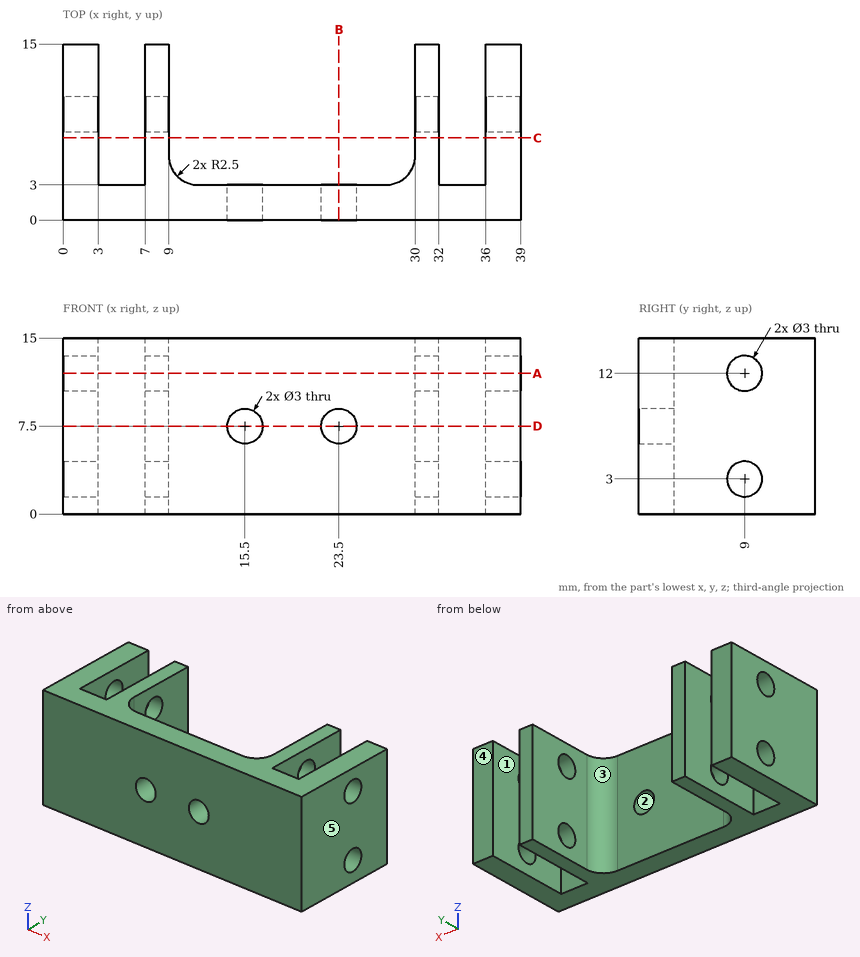
Could you check a few things on this drawing? It's one solid part, dimensions in mm from its lowest x, y, z. A direction names the side the tool comes from. Round coordinates to 2 decimals unless told otherwise and drop trailing zeros. Order: outer loops, then holes, each group sorted by start corner. A loop starts at its lowest first (then second) coordinate and runs counter-clockwise, first axis right, second up.
Q1. Please list where these lines run through material, in increasing order: probe 1 along X at (y, z) = (12.5, 3.75); probe 2 along X at (y, z) = (1.55, 7.5); probe 3 along Z at (x, y) = (7.6, 9).
Geometry says:
probe 1: x = 0 to 3, 7 to 9, 30 to 32, 36 to 39
probe 2: x = 0 to 14, 17 to 22, 25 to 39
probe 3: z = 0 to 1.5, 4.5 to 10.5, 13.5 to 15
Q2. Imagine slicing it at A-A, the plane z = 12. State how many separate pieces and enclosed holes the cut face has, then the cut area to 3 significant figures.
Geometry says:
separate pieces: 5
enclosed holes: 0
area: 210 mm2
Q3. Imagine slicing it at C-C, the plane y = 7. List the corners of the cut face in (x, z) for me.
Geometry says:
outline: (0, 0) - (3, 0) - (3, 15) - (0, 15) - close; (7, 0) - (9, 0) - (9, 15) - (7, 15) - close; (30, 0) - (32, 0) - (32, 15) - (30, 15) - close; (36, 0) - (39, 0) - (39, 15) - (36, 15) - close
Q4. Thinking about a two-plate mould opening in X: for the marked faces 3, 4 and 5, which applies, released by +X, released by -X, zero draft, split by the parting line, or undercut?
Geometry says:
face 3: undercut
face 4: zero draft
face 5: released by +X
Q5. Which directions (+Z, -Z, +X, -X, +Y, -Y) give clear straight access to the entire face, cutting with the end or side of a thin tool? Please do the marked faces 1 and 2.
Geometry says:
face 1: +Z, -Z, +Y
face 2: +Y, -Y
Q6. Imagine slicing it at D-D, the plane z = 7.5. List the corners of the cut face in (x, y) for me, then the cut area to 3 significant figures.
Geometry says:
outline: (0, 0) - (14, 0) - (14, 3) - (11.5, 3) arc R2.5 cw to (9, 5.5) - (9, 15) - (7, 15) - (7, 3) - (3, 3) - (3, 15) - (0, 15) - close; (17, 0) - (22, 0) - (22, 3) - (17, 3) - close; (25, 0) - (39, 0) - (39, 15) - (36, 15) - (36, 3) - (32, 3) - (32, 15) - (30, 15) - (30, 5.5) arc R2.5 cw to (27.5, 3) - (25, 3) - close
area: 222 mm2
Q7. I'm going to push flat-ended pins straight in: P1, Ø3, axis at x = 6.5, z = 10.5, coming from the -Y side; P2, Ø6, axis at x = 26, y = 6.5, coming from the -Z side; P3, Ø2, axis at x = 33.5, z = 10.5, coming from the +Y side. Where does each tip first touch, or does it pass through?
Geometry says:
P1: stops at y = 0
P2: passes through
P3: stops at y = 3
Q8. Imagine slicing it at B-B, the plane x = 23.5. List the corners of the cut face in (y, z) for me, then the cut area to 3 significant figures.
Geometry says:
outline: (0, 0) - (3, 0) - (3, 6) - (0, 6) - close; (0, 9) - (3, 9) - (3, 15) - (0, 15) - close
area: 36.0 mm2
